from build123d import *

# Parameters (mm, degrees)
F2_R = 1.979654
F3_R = 3.788583
F4_R = 1.653235
F5_R = 1.054441
F6_R = 1.312708
F7_R = 2.563491


with BuildPart() as f1:
    # F0 (on Front) → F1 (revolve)
    with BuildSketch(Plane.XZ):
        Polygon((-9.7125, 0), (0, 0), (0, 24.412502), (-9.1875, 24.412502), (-11.408553, 22.717658), (-14.042635, 22.871565), (-15.8375, 24.412502), (-19.512501, 24.412502), (-19.512501, 22.312501), (-10.4125, 19.6875), (-9.8875, 17.762501), (-12.5125, 8.4875), align=None)
    revolve(axis=Axis((0, 0, 12.206251), (0, 0, -1)))

    # F2
    f2_edges = [f1.edges().sort_by_distance(p)[0] for p in [
        (9.1875, 0, 24.412502),
    ]]
    fillet(f2_edges, radius=F2_R)

    # F3
    f3_edges = [f1.edges().sort_by_distance(p)[0] for p in [
        (14.042635, 0, 22.871565),
    ]]
    fillet(f3_edges, radius=F3_R)

    # F4
    f4_edges = [f1.edges().sort_by_distance(p)[0] for p in [
        (11.408553, 0, 22.717658),
    ]]
    fillet(f4_edges, radius=F4_R)

    # F5
    f5_edges = [f1.edges().sort_by_distance(p)[0] for p in [
        (15.8375, 0, 24.412502),
    ]]
    fillet(f5_edges, radius=F5_R)

    # F6
    f6_edges = [f1.edges().sort_by_distance(p)[0] for p in [
        (19.512501, 0, 22.312501),
    ]]
    fillet(f6_edges, radius=F6_R)

    # F7
    f7_edges = [f1.edges().sort_by_distance(p)[0] for p in [
        (12.5125, 0, 8.4875),
        (9.7125, 0, 0),
        (-11.1125, 0, 4.24375),
    ]]
    fillet(f7_edges, radius=F7_R)


solid = f1.part
Part model, mm, in its own coordinate system. A direction names the side the tool comes from. Coordinates: 2 decimals unless noted, no trailing zeros. Loops run counter-clockwise (first coordinate to the right, second up) from the corner with the lowest first, then second, coordinate; pieces in that order, holes last. Notation, with made-up numbers: (43.25, 9.5) - (87.25, 9.5) arc R33 ccw to (87.25, 41.5) - close; hole circle Ø5 at (49.5, -31.5). An arc over 180 degrees is marked (long way). Write each question's results on one line, items separated by ' | '. Start each with the question number.
Q1. Two-plate mould, pull along Z, no slides. Class faces 1 (the conical face through (-9.83, 3.1, 16.28)), 2 (the flat face through (0, 0, 24.413)), 3 (the conical face through (-9.91, 3.12, 2.05)): +Z half, -Z half, draft (parallel to the pull), parting line (faces both ways), or undercut.
Q2. Drop flat-ended pins along their axis: pin 1 Ø12 at (y, z) = (10, 6.5) entering from +X; pin 2 Ø12 at (y, z) = (-3.5, 17.5) entering from -X; pin 3 Ø4 at (x, y) = (-12.5, -2.5) entering from +Z. Give the stop position or say it passes through.
Q3. Which spindle directions (+Z, -Z, +X, -X, +Y, -Y) get a long thin tool onto all of the face, cutting with end or side? Do faces 4 (the conical face through (2.34, -10.55, 19.8)), 5 (the flat face through (-15, 7, 24.413)). Say none if no direction does.
Q4. Slice it at A-A on z = 5.5. Give the cut face in (x, y).
Q5. Slice it at B-B on z = 15.5. Give the cut face in (x, y), and give its area (3 significant figures).
Q6. Probe line 1 along Z through (x, y) = (-11, 15); line 2 along Z through (x, y) = (11, -16); line 3 along Y through (x, z) = (-9, 2.5). List the from-to ranges inside material, lowest first.
Answer:
1) face 1: undercut | face 2: +Z half | face 3: -Z half
2) pin 1: stops at x = 11.62 | pin 2: stops at x = -19.45 | pin 3: stops at z = 23.5
3) face 4: none | face 5: +Z, +X, -X, +Y, -Y
4) outline: circle Ø23.05 at (0, 0)
5) outline: circle Ø21.06 at (0, 0) | area: 348 mm2
6) line 1: z = 22.05 to 24.41 | line 2: z = 22.81 to 24.41 | line 3: y = -5.48 to 5.48
